Read the model definition and answer for the solid it produces. Units are mm, in the model's axes. Face numbers are marked on the shaded views. Give positions to 0.01 mm unless a question says otherwise; leave off trailing zeros. Order: outer loops, then holes, each group sorted by start corner. A loop starts at its lowest first (then second) coordinate and runs counter-clockwise, first axis right, second up. Notation, with made-up numbers: (74.5, -4.75) - (110.5, -4.75) arc R33 ccw to (110.5, 33.25) - close; hole circle Ø9 at (73.5, 79.25). An arc over 180 degrees is marked (long way). Write item = value, one per line.
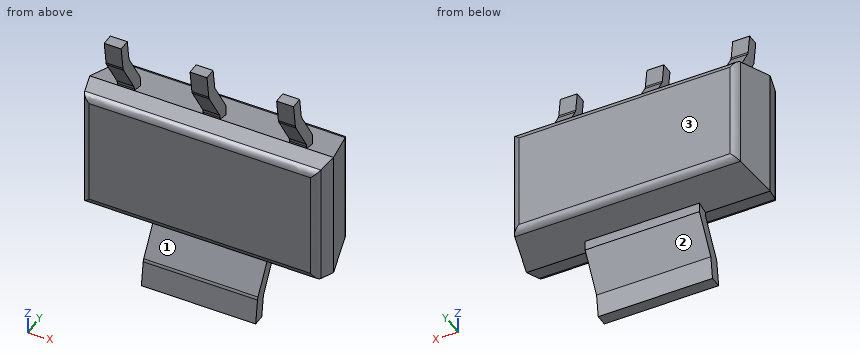
```python
from build123d import *

# Parameters (mm, degrees)
SKETCH5_W           = 6.505
SKETCH5_H           = 3.505
BOSS_EXTRUDE1_DEPTH = 1.2
BOSS_EXTRUDE1_TAPER = 13
SKETCH5_2_W         = 6.505
SKETCH5_2_H         = 3.505
BOSS_EXTRUDE2_DEPTH = 0.6
BOSS_EXTRUDE2_TAPER = 13
BOSS_EXTRUDE3_DEPTH = 0.226
BOSS_EXTRUDE4_DEPTH = 1.525
BOSS_EXTRUDE5_DEPTH = 0.226
BOSS_EXTRUDE6_DEPTH = 0.226
FILLET1_R           = 0.2
FILLET2_R           = 0.2


with BuildPart() as part:
    # Sketch5 → Boss-Extrude1 (new body)
    with BuildSketch(Plane(origin=(0, 0, 0), x_dir=(1, 0, 0), z_dir=(0, 1, 0))):
        Rectangle(SKETCH5_W, SKETCH5_H)
    extrude(amount=BOSS_EXTRUDE1_DEPTH, taper=BOSS_EXTRUDE1_TAPER)

    # Sketch5_2 → Boss-Extrude2 (add)
    with BuildSketch(Plane(origin=(0, 0, 0), x_dir=(1, 0, 0), z_dir=(0, 1, 0))):
        Rectangle(SKETCH5_2_W, SKETCH5_2_H)
    extrude(amount=-BOSS_EXTRUDE2_DEPTH, taper=BOSS_EXTRUDE2_TAPER)

    # Sketch6 → Boss-Extrude3 (add, symmetric)
    with BuildSketch(Plane(origin=(0, 0, 0), x_dir=(0, 0, -1), z_dir=(1, 0, 0))):
        Polygon((-2.903570514, -0.269279893), (-3.5, -0.35310259), (-3.5, -0.6611), (-2.8, -0.562721416), (-1.859056144, 0), (-1.7525, 0), (-1.682085202, 0.305), (-1.943299372, 0.305), align=None)
    boss_extrude3 = extrude(amount=BOSS_EXTRUDE3_DEPTH, both=True)

    # Mirror1: Boss-Extrude3 across plane
    add(boss_extrude3.mirror(Plane.XY))

    # Sketch7 → Boss-Extrude4 (add, symmetric)
    with BuildSketch(Plane(origin=(0, 0, 0), x_dir=(0, 0, -1), z_dir=(1, 0, 0))):
        Polygon((2.903570514, -0.269279893), (1.943299372, 0.305), (1.682085202, 0.305), (1.7525, 0), (1.859056144, 0), (2.8, -0.562721416), (3.5, -0.6611), (3.5, -0.35310259), align=None)
    extrude(amount=BOSS_EXTRUDE4_DEPTH, both=True)

    # Sketch8 → Boss-Extrude5 (add, symmetric)
    with BuildSketch(Plane.ZY.offset(2.29)):
        Polygon((1.859056144, 0), (2.8, -0.562721416), (3.5, -0.6611), (3.5, -0.35310259), (2.903570514, -0.269279893), (1.943299372, 0.305), (1.682085202, 0.305), (1.7525, 0), align=None)
    extrude(amount=BOSS_EXTRUDE5_DEPTH, both=True)

    # Sketch9 → Boss-Extrude6 (add, symmetric)
    with BuildSketch(Plane(origin=(2.31, 0, 0), x_dir=(0, 0, -1), z_dir=(1, 0, 0))):
        Polygon((-2.8, -0.562721416), (-1.859056144, 0), (-1.7525, 0), (-1.682085202, 0.305), (-1.943299372, 0.305), (-2.903570514, -0.269279893), (-3.5, -0.35310259), (-3.5, -0.6611), align=None)
    extrude(amount=BOSS_EXTRUDE6_DEPTH, both=True)

    # Fillet1
    fillet1_edges = [part.edges().sort_by_distance(p)[0] for p in [
        (-2.975458171, 1.2, 0),
        (0, 1.2, 1.475458171),
        (3.113979085, -0.6, 0),
        (0, -0.6, 1.613979085),
        (-3.113979085, -0.6, 0),
        (0, -0.6, -1.613979085),
        (2.975458171, 1.2, 0),
        (0, 1.2, -1.475458171),
    ]]
    fillet(fillet1_edges, radius=FILLET1_R)

    # Fillet2
    fillet2_edges = [part.edges().sort_by_distance(p)[0] for p in [
        (0, -0.562721416, -2.8),
        (0, 0, -1.859056144),
        (-2.29, -0.562721416, 2.8),
        (-2.29, 0, 1.859056144),
        (0, -0.562721416, 2.8),
        (0, 0, 1.859056144),
        (2.31, -0.562721416, 2.8),
        (2.31, 0, 1.859056144),
        (-2.29, 0.305, 1.943299372),
        (-2.29, -0.269279893, 2.903570514),
        (0, 0.305, 1.943299372),
        (0, -0.269279893, 2.903570514),
        (2.31, -0.269279893, 2.903570514),
        (2.31, 0.305, 1.943299372),
    ]]
    fillet(fillet2_edges, radius=FILLET2_R)


solid = part.part
```
1. Determine the mould class of the marked faces 1, 2 and 3 for opening direction Z: +Z half, -Z half, draft (parallel to the pull), parting line (faces both ways), or undercut.
Recorded:
face_1 = undercut
face_2 = -Z half
face_3 = draft
2. Section A-A (z = 2.25) is taken. Determine the outline of the cut face in (x, y).
Recorded:
outline = (-2.52, -0.23) - (-2.06, -0.23) - (-2.06, 0.12) - (-2.52, 0.12) - close; (-0.23, -0.23) - (0.23, -0.23) - (0.23, 0.12) - (-0.23, 0.12) - close; (2.08, -0.23) - (2.54, -0.23) - (2.54, 0.12) - (2.08, 0.12) - close
3. Section B-B (z = -2.5) is taken. Determine the outline of the cut face in (x, y) (3 decimals), and give its area (3 significant figures).
Recorded:
outline = (-1.525, -0.383) - (1.525, -0.383) - (1.525, -0.028) - (-1.525, -0.028) - close
area = 1.08 mm^2
4. Straight lines are drawn through the part: L1, parallel to X at y = -0.35, z = 3.25; L2, parallel to Z at x = -3, y = 0.45; L3, parallel to Y at x = 1.5, z = 0.5. For each, find the intervals that lie inside material, in ascending order. Write a range as [from, to].
Recorded:
L1 = [-2.52, -2.06], [-0.23, 0.23], [2.08, 2.54]
L2 = [-1.65, 1.65]
L3 = [-0.6, 1.2]
5. Flat-ended cylindrical pins translate along their axes: pin 1 (0.5 mm diameter, centred on y = -0.5, z = 2.5, fed in from -X); pin 2 (0.5 mm diameter, centred on y = 0, z = 3, fed in from -X); pin 3 (0.8 mm diameter, centred on y = 0, z = -2.5, fed in from +X) (3 decimals); pin 4 (0.8 mm diameter, centred on y = -0.5, z = 2, fed in from +X). Find the tip coordinate at first contact, or state that the pin passes through.
Recorded:
pin_1 = -2.52
pin_2 = through
pin_3 = 1.525
pin_4 = 3.2
